Geometry check sheet. Reference: the model listing, model coordinates, mm. Coordinates: 2 decimals unless noted, no trailing zeros. Order: outer loops, then holes, each group sorted by start corner. A loop starts at its lowest first (then second) coordinate and runs counter-clockwise, first axis right, second up. Notation, with made-up numbers: M 48,-2 L 92,-2 A16 cw 92,13 Z; hole C 11,-27.75 d3. An arc over 180 degrees is marked long. One line per item, written item: value. Start each with the question number.
1) Sectioned sample at B-B, the plane x = 44.5. Enter the section's corners in (y, z).
2) Thickness scan on L1, parallel to Y at x = 40, z = 1.8; L2, parallel to Y at x = 30, z = 2.2; L3, parallel to X at y = 40, z = 2.35. Record the ranges inside material, lowest first. Write a range as from..to.
3) Sectioned sample at D-D, the plane x = 13. Enter the section's corners in (y, z), then the cut area to 3 significant figures.
4) Go/stop test with flat-tipped pins: P1, Ø1.5, axis at y = 45.5, z = 2, coming from the -X side; P2, Ø0.9, axis at y = 41.5, z = 1.5, coming from the +X side; P3, Ø0.9, axis at x = 63, z = 2, coming from the -Y side. Record where each tip stops, or that it passes through.
5) Sectioned sample at A-A, the plane y = 31. Enter the section's corners in (x, z).
6) Sectioned sample at C-C, the plane z = 2. State how many separate pieces and enclosed holes the cut face has, then the cut area to 3 significant figures.
```python
from build123d import *

# Parameters (mm, degrees)
SKETCH2_R           = 8
SKETCH2_R_2         = 6
SKETCH2_W           = 7.6
SKETCH2_H           = 24.4
BOSS_EXTRUDE1_DEPTH = 3


with BuildPart() as part:
    # Sketch2 → Boss-Extrude1 (new body)
    with BuildSketch(Plane.XY):
        with BuildLine():
            Line((81.032103119, 50.181312), (81.032103119, 60.181312))
            Line((81.032103119, 60.181312), (78.032103119, 60.181312))
            Line((78.032103119, 60.181312), (78.032103119, 71.181312))
            ThreePointArc((78.032103119, 71.181312), (73.050090858, 72.33654353), (67.936161846, 72.284235691))
            ThreePointArc((67.936161846, 72.284235691), (62.235942644, 70.892785416), (56.438402104, 69.988818319))
            ThreePointArc((56.438402104, 69.988818319), (51.886102873, 69.971964975), (47.437133801, 70.93653043))
            ThreePointArc((47.437133801, 70.93653043), (41.102316828, 72.343050119), (34.613643935, 72.416041905))
            ThreePointArc((34.613643935, 72.416041905), (40.990344282, 77.154811793), (48.755286163, 78.83526559))
            ThreePointArc((48.755286163, 78.83526559), (48.80614848, 78.851120911), (48.85704212, 78.866875402))
            ThreePointArc((48.85704212, 78.866875402), (50.134187725, 81.487874692), (47.847872498, 83.297156554))
            ThreePointArc((47.847872498, 83.297156554), (24.351235249, 84.294658733), (3.641458375, 73.150507154))
            ThreePointArc((3.641458375, 73.150507154), (2.19654611, 59.548103084), (6.61028157, 46.600821237))
            ThreePointArc((6.61028157, 46.600821237), (6.138572184, 41.181312), (6.61028157, 35.761802763))
            ThreePointArc((6.61028157, 35.761802763), (2.19654611, 22.814520916), (3.641458375, 9.212116846))
            ThreePointArc((3.641458375, 9.212116846), (24.351235249, -1.932034733), (47.847872498, -0.934532554))
            ThreePointArc((47.847872498, -0.934532554), (50.134187725, 0.874749308), (48.85704212, 3.495748598))
            ThreePointArc((48.85704212, 3.495748598), (48.80614848, 3.511503089), (48.755286163, 3.52735841))
            ThreePointArc((48.755286163, 3.52735841), (40.990344282, 5.207812207), (34.613643935, 9.946582095))
            ThreePointArc((34.613643935, 9.946582095), (41.102316828, 10.019573881), (47.437133801, 11.42609357))
            ThreePointArc((47.437133801, 11.42609357), (51.886102873, 12.390659025), (56.438402104, 12.373805681))
            ThreePointArc((56.438402104, 12.373805681), (62.235942644, 11.469838584), (67.936161846, 10.078388309))
            ThreePointArc((67.936161846, 10.078388309), (73.050090858, 10.02608047), (78.032103119, 11.181312))
            Line((78.032103119, 11.181312), (78.032103119, 22.181312))
            Line((78.032103119, 22.181312), (81.032103119, 22.181312))
            Line((81.032103119, 22.181312), (81.032103119, 32.181312))
            Line((81.032103119, 32.181312), (78.032103119, 32.181312))
            Line((78.032103119, 32.181312), (78.032103119, 50.181312))
            Line((78.032103119, 50.181312), (81.032103119, 50.181312))
        make_face()
        with Locations((23.507028058, 53.931312)):
            Circle(SKETCH2_R, mode=Mode.SUBTRACT)
        with Locations((43.507028058, 41.181312)):
            Circle(SKETCH2_R_2, mode=Mode.SUBTRACT)
        with Locations((23.507028058, 28.431312)):
            Circle(SKETCH2_R, mode=Mode.SUBTRACT)
        with Locations((64.432028058, 41.181312)):
            Rectangle(SKETCH2_W, SKETCH2_H, mode=Mode.SUBTRACT)
    extrude(amount=BOSS_EXTRUDE1_DEPTH)


solid = part.part
```
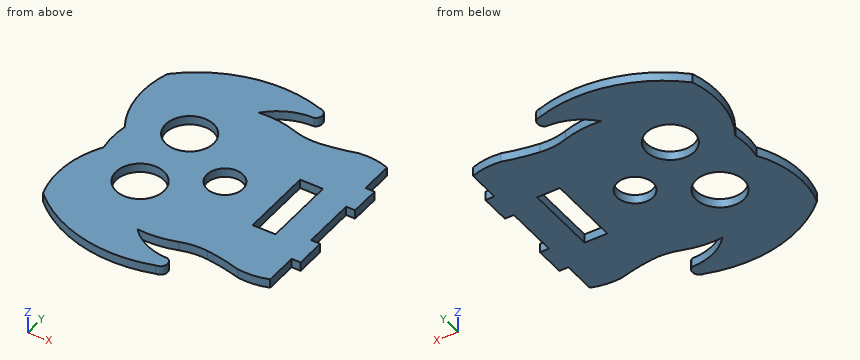
Final values:
1. outline: M -1.87,0 L 4.02,0 L 4.02,3 L -1.87,3 Z; M 10.6,0 L 35.26,0 L 35.26,3 L 10.6,3 Z; M 47.1,0 L 71.76,0 L 71.76,3 L 47.1,3 Z; M 78.35,0 L 84.23,0 L 84.23,3 L 78.35,3 Z
2. L1: y = -2.69..5.69, 9.91..36.31, 46.05..72.45, 76.67..85.05
2. L2: y = -2.85..23.76, 33.1..49.26, 58.6..85.21
2. L3: x = 6.16..37.62, 49.39..60.63, 68.23..78.03
3. outline: M 2.38,0 L 79.99,0 L 79.99,3 L 2.38,3 Z
3. area: 233 mm^2
4. P1: stops at x = 6.34
4. P2: stops at x = 78.03
4. P3: stops at y = 11.22
5. outline: M 4.24,0 L 15.93,0 L 15.93,3 L 4.24,3 Z; M 31.08,0 L 60.63,0 L 60.63,3 L 31.08,3 Z; M 68.23,0 L 81.03,0 L 81.03,3 L 68.23,3 Z
6. separate pieces: 1
6. enclosed holes: 4
6. area: 4,720 mm^2
